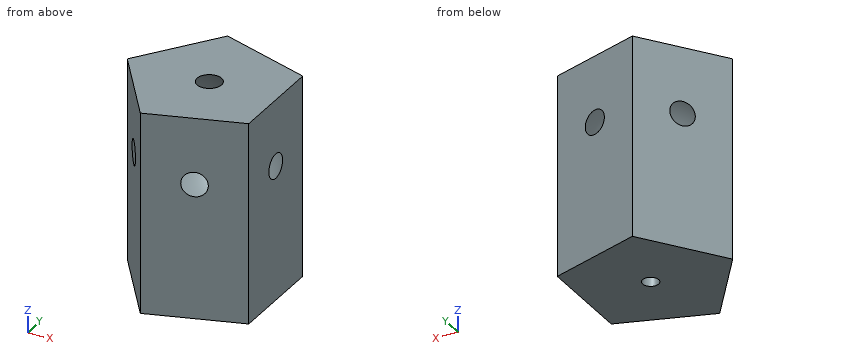
```python
from build123d import *

# Parameters (mm, degrees)
PAD_DEPTH    = 250
SKETCH001_R  = 10
POCKET_DEPTH = 250.001


with BuildPart() as obj1:
    # Sphere → Sphere (revolve)
    with BuildSketch(Plane(origin=(0, 0, 167.417), x_dir=(1, 0, 0), z_dir=(0, -1, 0))):
        with BuildLine():
            ThreePointArc((0, -83.9829), (83.9829, 0), (0, 83.9829))
            Line((0, 83.9829), (0, -83.9829))
        make_face()
    revolve(axis=Axis((0, 0, 167.417), (0, 0, 1)))


with BuildPart() as cut:
    # Sketch → Pad (new body)
    with BuildSketch(Plane.XY):
        Polygon((-31.543867, 97.082039), (-102.078097, 0), (-31.543867, -97.082039), (82.582915, -60), (82.582915, 60), align=None)
    extrude(amount=PAD_DEPTH)

    # Sketch001 → Pocket (cut, through all)
    with BuildSketch(Plane.XY.offset(250)):
        Circle(SKETCH001_R)
    extrude(amount=-POCKET_DEPTH, mode=Mode.SUBTRACT)

    # Cut: cut obj1
    add(obj1.part, mode=Mode.SUBTRACT)


solid = cut.part
```
CAD build for the part. Positions are in the model's coordinates, mm. Coordinates: 2 decimals unless noted, no trailing zeros. Order: outer loops, then holes, each group sorted by start corner. A loop starts at its lowest first (then second) coordinate and runs counter-clockwise, first axis right, second up. Notation, with made-up numbers: (54, -33) -> (71, -33) arc R10 ccw to (71, -16) -> close; hole circle Ø4 at (87, -11.5). An arc over 180 degrees is marked (long way). Use one line per item in the form item = value. Start each with the question number.
1) Band-saw the part on A-A on z = 179. Give the cut face in (x, y), then the cut area to 3 significant figures.
2) Band-saw the part on C-C on x = 0. Give the cut face in (y, z), then the cut area to 3 significant figures.
3) Band-saw the part on D-D on y = -72. Give the cut face in (x, z).
4) Drill centre lines: L1, parallel to X at y = 34.5, z = 194; L2, parallel to X at y = -14, z = 180; L3, parallel to Y at x = 56.5, z = 208.5. Where is each one in solid material? Low to high. Write a range as [from, to].
5) Drop flat-ended pins along their axis: pin 1 (3 mm diameter, centred on y = 57.5, z = 200, fed in from -X); pin 2 (4 mm diameter, centred on x = 23, z = 72, fed in from -Y). Give the stop position or say it passes through.
6) Band-saw the part on B-B on z = 63. Give the cut face in (x, y), then the cut area to 3 significant figures.
Entries:
q1.outline = (-102.08, 0) -> (-72.66, -40.49) arc R83.18 cw to (-72.66, 40.49) -> close; (-60.96, -56.59) -> (-31.54, -97.08) -> (16.06, -81.62) arc R83.18 cw to start; (-60.96, 56.59) arc R83.18 cw to (16.06, 81.62) -> (-31.54, 97.08) -> close; (34.98, -75.47) -> (82.58, -60) -> (82.58, -9.95) arc R83.18 cw to start; (34.98, 75.47) arc R83.18 cw to (82.58, 9.95) -> (82.58, 60) -> close
q1.area = 3,080 mm2
q2.outline = (-86.83, 0) -> (-10, 0) -> (-10, 84.03) arc R83.98 cw to (-15.27, 250) -> (-86.83, 250) -> close; (10, 0) -> (86.83, 0) -> (86.83, 250) -> (15.27, 250) arc R83.98 cw to (10, 84.03) -> close
q2.area = 19,600 mm2
q3.outline = (-49.77, 0) -> (45.65, 0) -> (45.65, 250) -> (-49.77, 250) -> close; hole circle Ø86.47 at (0, 167.42)
q4.L1 = [-77.01, -71.81], [71.81, 82.58]
q4.L2 = [-91.91, -81.85], [81.85, 82.58]
q4.L3 = [-68.47, -46.62], [46.62, 68.47]
q5.pin_1 = -61.39
q5.pin_2 = -80.01
q6.outline = (-102.08, 0) -> (-31.54, -97.08) -> (82.58, -60) -> (82.58, 60) -> (-31.54, 97.08) -> close; hole circle Ø20 at (0, 0)
q6.area = 24,500 mm2
